```python
from build123d import *

# Parameters (mm, degrees)
F0_R     = 0.4318
F0_R_2   = 0.4445
F1_DEPTH = 1.27
F3_DEPTH = 1.27


# Not quite as in the source:
# - ends of sketch curves that miss each other by under 0.0002 mm in the source are joined


with BuildPart() as f1:
    # F0 (on Top) → F1 (new body)
    with BuildSketch(Plane.XY):
        with BuildLine():
            Line((9.5249989071, 5.499263207), (-2.1858e-06, 10.9985226281))
            Line((-2.1858e-06, 10.9985226281), (-9.5250010929, 5.499259421))
            Line((-9.5250010929, 5.499259421), (-19.0459112442, 10.9961569369))
            ThreePointArc((-19.0459112442, 10.9961569369), (-21.4157534444, 11.6311591353), (-19.6809068475, 9.8963021357))
            Line((-19.6809068475, 9.8963021357), (-9.5250008015, 4.0327897373))
            Line((-9.5250008015, 4.0327897373), (-9.5249991985, -4.0327941963))
            Line((-9.5249991985, -4.0327941963), (-19.6850080876, -9.8986699867))
            ThreePointArc((-19.6850080876, -9.8986699867), (-21.4198613847, -11.6335212151), (-19.0500087433, -10.9985226281))
            Line((-19.0500087433, -10.9985226281), (-9.5249989071, -5.499263207))
            Line((-9.5249989071, -5.499263207), (2.1858e-06, -10.9985226281))
            Line((2.1858e-06, -10.9985226281), (9.5250010929, -5.499259421))
            Line((9.5250010929, -5.499259421), (9.5249991985, 4.0327941963))
            Line((9.5249991985, 4.0327941963), (19.0500087433, 9.5320534491))
            Line((19.0500087433, 9.5320534491), (28.5750185796, 4.0327940281))
            Line((28.5750185796, 4.0327940281), (38.1000284158, 9.5320534491))
            Line((38.1000284158, 9.5320534491), (46.9900389078, 4.3994105656))
            Line((46.9900389078, 4.3994105656), (47.625038252, 5.499263207))
            Line((47.625038252, 5.499263207), (39.3991596309, 10.2484699041))
            Line((39.3991596309, 10.2484699041), (39.3991596309, 10.224751758))
            Line((39.3991596309, 10.224751758), (38.673771624, 10.6672722885))
            Line((38.673771624, 10.6672722885), (38.1000284158, 10.9985226281))
            Line((38.1000284158, 10.9985226281), (37.6488161101, 10.7380154406))
            Line((37.6488161101, 10.7380154406), (37.6488161101, 10.731614756))
            Line((37.6488161101, 10.731614756), (36.7598161101, 10.224751758))
            Line((36.7598161101, 10.224751758), (28.5750185796, 5.499263207))
            Line((28.5750185796, 5.499263207), (19.6850087433, 10.6319053096))
            Line((19.6850087433, 10.6319053096), (19.6850087433, 10.9985226281))
            Line((19.6850087433, 10.9985226281), (19.6850087433, 21.9970528281))
            ThreePointArc((19.6850087433, 21.9970528281), (19.0500083949, 24.3669048897), (18.4150080465, 21.9970528281))
            Line((18.4150080465, 21.9970528281), (18.4150080465, 10.9985226281))
            Line((18.4150080465, 10.9985226281), (18.4150080465, 10.6319053096))
            Line((18.4150080465, 10.6319053096), (9.5249989071, 5.499263207))
        make_face()
        with Locations((-20.3200087433, -10.9985218709)):
            Circle(F0_R, mode=Mode.SUBTRACT)
        Polygon((8.2550007723, -3.8861430213), (8.2550009472, -4.7660248316), (1.8944e-06, -9.5320529443), (-0.761998193, -9.0921121906), align=None, mode=Mode.SUBTRACT)
        Polygon((-8.255, -1.6406e-06), (-8.2550009472, 4.7660248316), (-7.493, 5.2059664855), (-7.493, -1.6406e-06), (-7.493, -5.2059682691), (-8.2549990528, -4.7660281127), align=None, mode=Mode.SUBTRACT)
        Polygon((-6.604, -5.499263207), (-6.604, 5.7192311104), (-1.6510017049, 8.5788473218), (8.2549994317, 2.8596175239), (8.2550005683, -2.8596142427), (-1.6509982951, -8.578847978), (-6.604, -5.7192324228), align=None, mode=Mode.SUBTRACT)
        with Locations((-20.3159024508, 10.9961569369)):
            Circle(F0_R_2, mode=Mode.SUBTRACT)
        Polygon((-1.8944e-06, 9.5320529443), (8.2549990528, 4.7660281127), (8.2549992277, 3.8861463025), (-0.762001807, 9.0921118878), align=None, mode=Mode.SUBTRACT)
        with Locations((19.0500083949, 23.0969048897)):
            Circle(F0_R_2, mode=Mode.SUBTRACT)
        Polygon((36.7598161101, 10.731614756), (36.7598161101, 10.224751758), (37.6488161101, 10.7380154406), (37.6488161101, 11.8624546668), (38.5683002365, 10.731614756), (38.673771624, 10.6672722885), (39.3991596309, 10.2484699041), (39.3991596309, 10.731614756), (39.3991596309, 13.271614756), (38.5101596309, 13.271614756), (38.5101596309, 12.0436610678), (37.6488161101, 13.271614756), (36.7598161101, 13.271614756), align=None)
        Polygon((37.6488161101, 10.7380154406), (36.7598161101, 10.224751758), (37.6488161101, 10.731614756), align=None)
        Polygon((39.3991596309, 10.2484699041), (38.673771624, 10.6672722885), (39.3991596309, 10.224751758), align=None)
    extrude(amount=F1_DEPTH)

    # F2 (on Top) → F3 (join)
    with BuildSketch(Plane.XY):
        Polygon((37.6677321614, 13.1759580532), (36.7787321614, 13.1759580532), (36.7787321614, 10.6359580532), (36.7787321614, 10.1290950552), (37.6677321614, 10.6359580532), (37.6677321614, 11.7667979639), (38.5872162879, 10.6359580532), (39.4180756822, 10.1290950552), (39.4180756822, 10.6359580532), (39.4180756822, 13.1759580532), (38.5290756822, 13.1759580532), (38.5290756822, 11.948004365), align=None)
    extrude(amount=F3_DEPTH)


solid = f1.part
```
Check sheet for the modelled part. Datum: model origin and axes. Units: mm. A direction names the side the tool comes from. Coordinates: 2 decimals unless noted, no trailing zeros. Write each loop counter-clockwise with the first axis right and the second up, starting at its lowest first coordinate (ties: lowest second). Pieces come first, ordered by that corner, then holes. Notation, with made-up numbers: (66, 6.5) - (80, 6.5) arc R27 ccw to (80, 36.5) - close; hole circle Ø7 at (64, 29.5). An arc over 180 degrees is marked (long way). One line per question, with ' | ' between items.
Item 1: Sectioned sample at C-C on x = -12. Record the boundary of the cut face in (y, z), plus the area to 3 significant figures.
Determined:
outline: (-6.93, 0) - (-5.46, 0) - (-5.46, 1.27) - (-6.93, 1.27) - close; (5.46, 0) - (6.93, 0) - (6.93, 1.27) - (5.46, 1.27) - close | area: 3.72 mm2
Item 2: Mould release check, pull along X, two halves, no side actions. Record for faces 4 (the face through (43.579, 7.835, 0.626)), 5 (the face through (19.097, 24.366, 0.626)), 6 (the face through (42.483, 7.002, 0.626)): pulls with the +X half, pulls with the -X half, needs draft (parallel to the pull), parting line crosses it, or undercut.
Determined:
face 4: pulls with the +X half | face 5: parting line crosses it | face 6: undercut
Item 3: Sectioned sample at A-A on y = 0. Record the boundary of the cut face in (x, z) (3 decimals), plus the area to 3 significant figures.
Determined:
outline: (-9.525, 0) - (-8.255, 0) - (-8.255, 1.27) - (-9.525, 1.27) - close; (-7.493, 0) - (-6.604, 0) - (-6.604, 1.27) - (-7.493, 1.27) - close; (8.255, 0) - (9.525, 0) - (9.525, 1.27) - (8.255, 1.27) - close | area: 4.35 mm2
Item 4: Gauge pin test, flat ends, axial feed: P1, Ø12, axis at x = 29.5, y = -6.5, coming from the +Z side; P2, Ø0.6, axis at y = 1, z = 0.5, coming from the +X side (3 decimals); P3, Ø0.6, axis at y = 14, z = 1, coming from the -X side (3 decimals). Record the tip position at first contact, or that the pin passes through.
Determined:
P1: passes through | P2: stops at x = 9.525 | P3: stops at x = 18.415
Item 5: Thickness scan on line 1 (X direction, y = -4, z = 0.35) (3 decimals); line 2 (X direction, y = -8, z = 0.35); line 3 (X direction, y = -3, z = 0.95) (3 decimals). Record the ranges inside material, lowest first. Write a range as [from, to].
Determined:
line 1: x = [-9.525, -8.255], [-7.493, -6.604], [6.28, 8.058], [8.255, 9.525] | line 2: x = [-16.4, -13.86], [-5.19, -2.65], [-0.65, 1.13], [2.65, 5.19] | line 3: x = [-9.525, -8.255], [-7.493, -6.604], [8.012, 9.525]
Item 6: Sectioned sample at D-D on y = 16. Record the boundary of the cut face in (x, z) (3 decimals).
Determined:
outline: (18.415, 0) - (19.685, 0) - (19.685, 1.27) - (18.415, 1.27) - close
Item 7: Sectioned sample at B-B on x = 4. Record the boundary of the cut face in (y, z), plus the area to 3 significant figures.
Determined:
outline: (-8.69, 0) - (-7.22, 0) - (-7.22, 1.27) - (-8.69, 1.27) - close; (-6.34, 0) - (-5.32, 0) - (-5.32, 1.27) - (-6.34, 1.27) - close; (5.32, 0) - (6.34, 0) - (6.34, 1.27) - (5.32, 1.27) - close; (7.22, 0) - (8.69, 0) - (8.69, 1.27) - (7.22, 1.27) - close | area: 6.33 mm2
Item 8: Access from +Z, -Z, +X, -X, +Y, -Y to the whole of each face (thin tool, end or side, straight path). Record for faces 1 (the face through (9.525, -1, 1)), 2 (the face through (-4.16, 7.13, 0.63)), 3 (the face through (4.83, 8.21, 0.63)).
Determined:
face 1: +Z, -Z, +X, -Y | face 2: +Z, -Z | face 3: +Z, -Z, +Y
